```python
from build123d import *

# Parameters (mm, degrees)
BOSS_EXTRUDE1_DEPTH      = 76.2
BOSS_EXTRUDE1_DEPTH_BACK = 76.2
SKETCH3_W                = 76.2
SKETCH3_H                = 50.8
SKETCH3_W_2              = 69.85
SKETCH3_H_2              = 44.45
CUT_EXTRUDE1_DEPTH       = 100.190170884
CUT_EXTRUDE1_DEPTH_BACK  = 100.190170884
SKETCH7_R                = 4
CUT_EXTRUDE2_DEPTH       = 111.716033166
FILLET1_R                = 12.7


with BuildPart() as part:
    # Sketch3 → Boss-Extrude1 (new, two sides: drawn at the far end of the back side and taken through both)
    with BuildSketch(Plane.XY.offset(-BOSS_EXTRUDE1_DEPTH_BACK)):
        Rectangle(SKETCH3_W, SKETCH3_H)
        Rectangle(SKETCH3_W_2, SKETCH3_H_2, mode=Mode.SUBTRACT)
    extrude(amount=BOSS_EXTRUDE1_DEPTH + BOSS_EXTRUDE1_DEPTH_BACK)

    # Sketch6 → Cut-Extrude1 (cut, two sides: drawn at the far end of the back side and taken through both)
    with BuildSketch(Plane(origin=(0, 25.4, 0), x_dir=(1, 0, 0), z_dir=(0, 1, 0)).offset(-CUT_EXTRUDE1_DEPTH_BACK)):
        with BuildLine():
            Line((34.925, 76.2), (-34.925, 76.2))
            Line((-34.925, 76.2), (-34.925, -28.575))
            ThreePointArc((-34.925, -28.575), (0, -63.5), (34.925, -28.575))
            Line((34.925, -28.575), (34.925, 76.2))
        make_face()
    extrude(amount=CUT_EXTRUDE1_DEPTH + CUT_EXTRUDE1_DEPTH_BACK, mode=Mode.SUBTRACT)

    # Sketch7 → Cut-Extrude2 (cut, through all)
    with BuildSketch(Plane(origin=(38.1, 0, 0), x_dir=(0, 0, -1), z_dir=(1, 0, 0))):
        with Locations((63.5, 0)):
            Circle(SKETCH7_R)
    extrude(amount=-CUT_EXTRUDE2_DEPTH, mode=Mode.SUBTRACT)

    # Fillet1
    fillet1_edges = [part.edges().sort_by_distance(p)[0] for p in [
        (36.5125, 25.4, -76.2),
        (-36.5125, -25.4, -76.2),
        (-36.5125, 25.4, -76.2),
        (36.5125, -25.4, -76.2),
    ]]
    fillet(fillet1_edges, radius=FILLET1_R)


solid = part.part
```
The model under review builds one solid part; all positions refer to its coordinate system, in mm. A direction names the side the tool comes from. Give positions to 0.01 mm unless a question says otherwise; leave off trailing zeros. Write each loop counter-clockwise with the first axis right and the second up, starting at its lowest first coordinate (ties: lowest second). Pieces come first, ordered by that corner, then holes. Notation, with made-up numbers: (71, -24.5) -> (75, -24.5) arc R28 cw to (75, -6.5) -> close; hole circle Ø11 at (-9, 47.25). An arc over 180 degrees is marked (long way). Answer in a Markdown table with one row per item.
1) Add section D-D on z = 49.5. State the section outline as (x, y) points (3 decimals), plus the area to 3 significant figures.
Worked answers:
| item | result |
|---|---|
| outline | (-38.1, -25.4) -> (-27.962, -25.4) -> (-27.962, -22.225) -> (-34.925, -22.225) -> (-34.925, 22.225) -> (-27.962, 22.225) -> (-27.962, 25.4) -> (-38.1, 25.4) -> close; (27.962, -25.4) -> (38.1, -25.4) -> (38.1, 25.4) -> (27.962, 25.4) -> (27.962, 22.225) -> (34.925, 22.225) -> (34.925, -22.225) -> (27.962, -22.225) -> close |
| area | 411 mm² |
2) For L1, parallel to X at y = 0, z = -52.5 (3 decimals); L2, parallel to Y at x = 36, z = -63, list the stretches that pass through material, from the lowest coordinate up. Write a range as [from, to].
Worked answers:
| item | result |
|---|---|
| L1 | [-38.1, -34.925], [34.925, 38.1] |
| L2 | [-25.4, -3.97], [3.97, 25.4] |
3) Add section A-A on x = 0. State the section outline as (y, z) points (3 decimals).
Worked answers:
| item | result |
|---|---|
| outline | (-25.4, 63.5) -> (-22.225, 63.5) -> (-22.225, 76.2) -> (-25.4, 76.2) -> close; (22.225, 63.5) -> (25.4, 63.5) -> (25.4, 76.2) -> (22.225, 76.2) -> close |
4) Mouldability with a two-part tool opening along X and no side actions: class faces 3 (the flat face through (38.1, 0, -1)), 4 (the flat face through (-9, -25.4, 63)), 5 (the flat face through (0, 22.225, 68)), 6 (the flat face through (-34.925, 0, -1)) as +X half, -X half, draft (parallel to the pull), parting line (faces both ways), or undercut.
Worked answers:
| item | result |
|---|---|
| face 3 | +X half |
| face 4 | draft |
| face 5 | undercut |
| face 6 | undercut |
5) Tool access review of faces 1 (the flat face through (0, -22.225, 68)), 2 (the cylindrical face through (36.535, -1.532, -67.195)): name each direction out of +Z, -Z, +X, -X, +Y, -Y from which nothing blocks a thin tool from reaching the whole face with its end or side.
Worked answers:
| item | result |
|---|---|
| face 1 | +Z, -Z |
| face 2 | +X, -X |
6) Clearance check with a flat-ended pin moving along its axis: P1, Ø14.5, axis at x = -3, z = 51.5, coming from the +Y side. State where the tip first meets the part, or that it passes through.
Worked answers:
| item | result |
|---|---|
| P1 | through |
7) Add section C-C on y = 0. State the section outline as (x, z) points (3 decimals), plus the area to 3 significant figures.
Worked answers:
| item | result |
|---|---|
| outline | (-38.1, -76.2) -> (-34.925, -76.2) -> (-34.925, -67.5) -> (-38.1, -67.5) -> close; (-38.1, -59.5) -> (-34.925, -59.5) -> (-34.925, 76.2) -> (-38.1, 76.2) -> close; (34.925, -76.2) -> (38.1, -76.2) -> (38.1, -67.5) -> (34.925, -67.5) -> close; (34.925, -59.5) -> (38.1, -59.5) -> (38.1, 76.2) -> (34.925, 76.2) -> close |
| area | 917 mm² |
8) Add section B-B on z = -28. State the section outline as (x, y) points (3 decimals).
Worked answers:
| item | result |
|---|---|
| outline | (-38.1, -25.4) -> (-34.925, -25.4) -> (-34.925, 25.4) -> (-38.1, 25.4) -> close; (34.925, -25.4) -> (38.1, -25.4) -> (38.1, 25.4) -> (34.925, 25.4) -> close |
